Check sheet for the modelled part. Datum: model origin and axes. Units: mm. Face numbers are marked on the shaded views. Round coordinates to 2 decimals unless told otherwise and drop trailing zeros. Order: outer loops, then holes, each group sorted by start corner. A loop starts at its lowest first (then second) coordinate and runs counter-clockwise, first axis right, second up.
Q1. Cross-section at D-D on x = -14. Record the cut outline in (y, z) (3 decimals), then the cut area to 3 significant figures.
Q2. Cross-section at C-C on y = 9. Record the cut outline in (x, z) (3 decimals).
Q3. Mould release check, pull along X, two halves, no side actions. Record for the marked faces 1, 2 and 3: +X half, -X half, draft (parallel to the pull), parting line (faces both ways), or undercut.
Q4. Cross-section at A-A on y = 0. Record the cut outline in (x, z) (3 decimals).
Q5. Scan lines: probe 1 along Y at (x, z) = (0, 2) (3 decimals); probe 2 along Z at (x, y) = (6, -15); probe 3 along Y at (x, z) = (16.5, 15.5). Record each from-to range of solid material in increasing order.
Q6. Depth check by flat-ended pin: P1, Ø4, axis at x = 0, y = 0, coming from the -Z side; P2, Ø1, axis at x = -11, z = 14.5, coming from the +Y side; P3, Ø1.5, axis at x = -12, z = 17, coming from the -Y side; P4, Ø5, axis at x = -16, y = 16.5, coming from the +Z side. Enter the tip coordinate at first touch or a pass-through.
from build123d import *

# Parameters (mm, degrees)
SKETCH1_R           = 28.575
BOSS_EXTRUDE1_DEPTH = 5.08
SKETCH2_R           = 3.175
BOSS_EXTRUDE2_DEPTH = 43.815
SKETCH6_R           = 3.175
CUT_EXTRUDE2_DEPTH  = 49.895


with BuildPart() as part:
    # Sketch1 → Boss-Extrude1 (new body)
    with BuildSketch(Plane.XY):
        Circle(SKETCH1_R)
    extrude(amount=BOSS_EXTRUDE1_DEPTH)

    # Sketch2 → Boss-Extrude2 (add)
    with BuildSketch(Plane.XY.offset(5.08)):
        with Locations((-18.542, 11.1125)):
            Circle(SKETCH2_R)
        with Locations((18.542, 11.1125)):
            Circle(SKETCH2_R)
        with Locations((-12.7, -14.125569529)):
            Circle(SKETCH2_R)
        with Locations((12.7, -14.125569529)):
            Circle(SKETCH2_R)
    extrude(amount=BOSS_EXTRUDE2_DEPTH)

    # Sketch6 → Cut-Extrude2 (cut, through all)
    with BuildSketch(Plane(origin=(0, 0, 0), x_dir=(-1, 0, 0), z_dir=(0, 0, -1))):
        Circle(SKETCH6_R)
    extrude(amount=-CUT_EXTRUDE2_DEPTH, mode=Mode.SUBTRACT)


solid = part.part
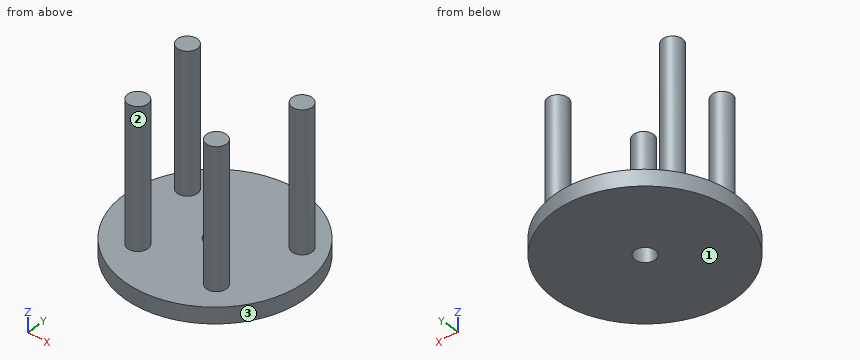
Results found:
1. outline: (-24.91, 0) - (24.91, 0) - (24.91, 5.08) - (-11.229, 5.08) - (-11.229, 48.895) - (-17.022, 48.895) - (-17.022, 5.08) - (-24.91, 5.08) - close
1. area: 507 mm2
2. outline: (-27.121, 0) - (27.121, 0) - (27.121, 5.08) - (20.912, 5.08) - (20.912, 48.895) - (16.172, 48.895) - (16.172, 5.08) - (-16.172, 5.08) - (-16.172, 48.895) - (-20.912, 48.895) - (-20.912, 5.08) - (-27.121, 5.08) - close
3. face 1: draft
3. face 2: undercut
3. face 3: parting line
4. outline: (-28.575, 0) - (-3.175, 0) - (-3.175, 5.08) - (-28.575, 5.08) - close; (3.175, 0) - (28.575, 0) - (28.575, 5.08) - (3.175, 5.08) - close
5. probe 1: y = -28.575 to -3.175, 3.175 to 28.575
5. probe 2: z = 0 to 5.08
5. probe 3: y = 8.68 to 13.54
6. P1: passes through
6. P2: stops at y = -11.19
6. P3: stops at y = -17.3
6. P4: stops at z = 5.08
